For this review, take the finished solid that the model builds, in its own axes (mm). Face numbers are marked on the shaded views. A direction names the side the tool comes from. Round coordinates to 2 decimals unless told otherwise and drop trailing zeros. Loops run counter-clockwise (first coordinate to the right, second up) from the corner with the lowest first, then second, coordinate; pieces in that order, holes last.
1) Take a section at A-A (z = 47). State the section outline as (x, y) points, then the cut area to 3 significant figures.
2) Take a section at C-C (y = -55.5). State the section outline as (x, z) points.
3) Take a section at D-D (x = 13.5). State the section outline as (y, z) points.
4) Tool access review of the marked faces 4, 5 and 6: name each direction out of +Z, -Z, +X, -X, +Y, -Y from which nothing blocks a thin tool from reaching the whole face with its end or side.
5) Wall thickness on L1, parallel to Z at x = 9.5, y = -69; L2, parallel to Y at x = 31, z = 49; L3, parallel to Z at x = 20, y = -51.75: over which ranges is each line inside the solid? List them lowest first.
6) Mouldability with a two-part tool opening along X and no side actions: class the marked faces 1, 2 and 3 as pulls with the +X half, pulls with the -X half, needs draft (parallel to the pull), parting line crosses it, or undercut.
7) Insertion check: pin 1 (3 mm diameter, centred on x = 10, y = -61, fed in from +Z); pin 2 (6.5 mm diameter, centred on x = 34.5, z = 39.5, fed in from -Y); pin 3 (4 mm diameter, centred on x = 22, y = -53.5, fed in from +Z). Each pin has a flat end and moves straight along its axis. Give the tip position at first contact, or say it passes through.
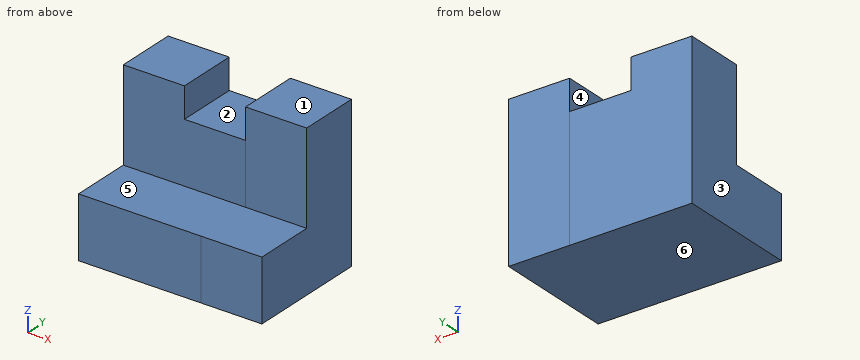
```python
from build123d import *

# Parameters (mm, degrees)
F1_DEPTH = 25.4
F2_DEPTH = 12.7
F3_W     = 12.7
F3_H     = 6.35
F4_DEPTH = 12.701


with BuildPart() as f1:
    # F0 (on Right) → F1 (new body)
    with BuildSketch(Plane.YZ):
        Polygon((-45.853703, 51.307991), (-58.553703, 51.307991), (-58.553703, 32.257991), (-71.253703, 32.257991), (-71.253703, 19.557991), (-45.853703, 19.557991), align=None)
    extrude(amount=F1_DEPTH)

    # F1_face (on face) → F2 (join)
    with BuildSketch(Plane(origin=(25.4, -55.832275, 32.711562), x_dir=(0, 1, 0), z_dir=(1, 0, 0))):
        Polygon((9.978571, 18.596429), (-2.721429, 18.596429), (-2.721429, -0.453571), (-15.421429, -0.453571), (-15.421429, -13.153571), (9.978571, -13.153571), align=None)
    extrude(amount=F2_DEPTH)

    # F3 (on face) → F4 (cut, through all)
    with BuildSketch(Plane.XZ.offset(58.553703)):
        with Locations((19.05, 48.132991)):
            Rectangle(F3_W, F3_H)
    extrude(amount=-F4_DEPTH, mode=Mode.SUBTRACT)


solid = f1.part
```
Response:
1. outline: (0, -58.55) - (12.7, -58.55) - (12.7, -45.85) - (0, -45.85) - close; (25.4, -58.55) - (38.1, -58.55) - (38.1, -45.85) - (25.4, -45.85) - close
1. area: 323 mm2
2. outline: (0, 19.56) - (38.1, 19.56) - (38.1, 51.31) - (25.4, 51.31) - (25.4, 44.96) - (12.7, 44.96) - (12.7, 51.31) - (0, 51.31) - close
3. outline: (-71.25, 19.56) - (-45.85, 19.56) - (-45.85, 44.96) - (-58.55, 44.96) - (-58.55, 32.26) - (-71.25, 32.26) - close
4. face 4: +Z, +Y, -Y
4. face 5: +Z, +X, -X, -Y
4. face 6: -Z, +X, -X, +Y, -Y
5. L1: z = 19.56 to 32.26
5. L2: y = -58.55 to -45.85
5. L3: z = 19.56 to 44.96
6. face 1: needs draft
6. face 2: undercut
6. face 3: pulls with the -X half
7. pin 1: stops at z = 32.26
7. pin 2: stops at y = -58.55
7. pin 3: stops at z = 44.96
